```python
from build123d import *

# Parameters (mm, degrees)
F0_R     = 3.15
F1_DEPTH = 1.2
F2_R     = 1


with BuildPart() as f1:
    # F0 (on Top) → F1 (new body)
    with BuildSketch(Plane.XY):
        Polygon((0, 25), (0, 0), (25, 0), (55, 0), (70, 0), (70, 25), (55, 25), (25, 25), align=None)
        with Locations((12.5, 12.5)):
            Circle(F0_R, mode=Mode.SUBTRACT)
        with Locations((40, 12.5)):
            Circle(F0_R, mode=Mode.SUBTRACT)
        with BuildLine():
            ThreePointArc((65.65, 11), (62.5, 7.85), (59.35, 11))
            Line((59.35, 11), (59.35, 14))
            ThreePointArc((59.35, 14), (62.5, 17.15), (65.65, 14))
            Line((65.65, 14), (65.65, 11))
        make_face(mode=Mode.SUBTRACT)
        Polygon((25, 0), (0, 0), (25, -30), align=None)
        Polygon((25, 55), (0, 25), (25, 25), align=None)
        Polygon((70, 0), (55, 0), (55, -20), align=None)
        Polygon((55, 45), (55, 25), (70, 25), align=None)
    extrude(amount=F1_DEPTH)

    # F2
    f2_edges = [f1.edges().sort_by_distance(p)[0] for p in [
        (0, 25, 0.6),
        (0, 0, 0.6),
        (70, 0, 0.6),
        (70, 25, 0.6),
    ]]
    fillet(f2_edges, radius=F2_R)


solid = f1.part
```
Here's how the part is built. I have some questions about the finished solid (model axes, mm). A direction names the side the tool comes from. Coordinates: 2 decimals unless noted, no trailing zeros. Order: outer loops, then holes, each group sorted by start corner. A loop starts at its lowest first (then second) coordinate and runs counter-clockwise, first axis right, second up. Notation, with made-up numbers: M 16.25,12.25 L 57.25,12.25 A22 cw 57.25,19.25 Z; hole C -25.5,-25 d9. An arc over 180 degrees is marked long. Answer as a JSON object with one key per item and string values. Group by question number.
(1) For pin 1 (0.6 mm diameter, centred on y = 34.5, z = 0.5, fed in from +X), with a flat end and sliding along its axis, tell me the tip position at first contact or that it passes through.
(2) If we mould it in two halves opening along Y, with no side actions, what happens to faces 1 (the face through (35, 13, 1.2)), 2 (the face through (62.57, 7.85, 0.59)), 3 (the face through (12.44, -14.93, 0.59))? For each: released by +Y, released by -Y, zero draft, split by the parting line, or undercut.
(3) I need wall thicknesses on probe 1 along X at (y, z) = (14, 0.6); probe 2 along Y at (x, z) = (40, 0.3); probe 3 along Y at (x, z) = (54, 0.85). Which ranges of each line are inside material? Lowest first, please.
(4) Which directions (+Z, -Z, +X, -X, +Y, -Y) give clear straight access to the entire face, cutting with the end or side of a thin tool? Please do faces 4 (the face through (62.43, 17.15, 0.59)), 5 (the face through (62.5, 35, 0.6)).
(5) Suppose I cut it at B-B, the plane y = 12.5. Please give me the cut outline in (x, z), then the cut area to 3 significant figures.
(6) Suppose I cut it at A-A, the plane x = 40. Please give me the cut outline in (y, z), then the cut area to 3 significant figures.
(7) Suppose I cut it at D-D, the plane y = -6. Please give me the cut outline in (x, z), then the cut area to 3 significant figures.
(8) Suppose I cut it at C-C, the plane z = 0.85. Please give me the cut outline in (x, y), then the cut area to 3 significant figures.
Values found:
{
 "1": {"pin 1": "stops at x = 63.1"},
 "2": {"face 1": "zero draft", "face 2": "undercut", "face 3": "released by -Y"},
 "3": {"probe 1": "x = 0 to 9.73, 15.27 to 37.23, 42.77 to 59.35, 65.65 to 70", "probe 2": "y = 0 to 9.35, 15.65 to 25", "probe 3": "y = 0 to 25"},
 "4": {"face 4": "+Z, -Z", "face 5": "+Z, -Z, +X, +Y"},
 "5": {"outline": "M 0,0 L 9.35,0 L 9.35,1.2 L 0,1.2 Z; M 15.65,0 L 36.85,0 L 36.85,1.2 L 15.65,1.2 Z; M 43.15,0 L 59.35,0 L 59.35,1.2 L 43.15,1.2 Z; M 65.65,0 L 70,0 L 70,1.2 L 65.65,1.2 Z", "area": "61.3 mm^2"},
 "6": {"outline": "M 0,0 L 9.35,0 L 9.35,1.2 L 0,1.2 Z; M 15.65,0 L 25,0 L 25,1.2 L 15.65,1.2 Z", "area": "22.4 mm^2"},
 "7": {"outline": "M 5,0 L 25,0 L 25,1.2 L 5,1.2 Z; M 55,0 L 65.5,0 L 65.5,1.2 L 55,1.2 Z", "area": "36.6 mm^2"},
 "8": {"outline": "M 0,0.36 A1 ccw 0.23,-0.28 L 25,-30 L 25,0 L 55,0 L 55,-20 L 69.8,-0.27 A1 ccw 70,0.33 L 70,24.67 A1 ccw 69.8,25.27 L 55,45 L 55,25 L 25,25 L 25,55 L 0.23,25.28 A1 ccw 0,24.64 Z; hole C 12.5,12.5 d6.3; hole C 40,12.5 d6.3; hole M 59.35,11 A3.15 ccw 65.65,11 L 65.65,14 A3.15 ccw 59.35,14 Z", "area": "2,690 mm^2"}
}
